Here's how the part is built. I have some questions about the finished solid (model axes, mm). Coordinates: 2 decimals unless noted, no trailing zeros. Write each loop counter-clockwise with the first axis right and the second up, starting at its lowest first coordinate (ties: lowest second). Pieces come first, ordered by that corner, then holes. Notation, with made-up numbers: (33, 8) -> (63, 8) arc R7 ccw to (63, 13) -> close; hole circle Ø2 at (51, -12.5). An arc over 180 degrees is marked (long way). Use CSV: the item, a comma, the result in double quotes. Start each with the question number.
```python
from build123d import *

# Parameters (mm, degrees)
CUT_EXTRUDE1_DEPTH = 0.8
FILLET1_R          = 0.1
FILLET2_R          = 0.1


with BuildPart() as part:
    # Sketch1 → Revolve1 (revolve)
    with BuildSketch(Plane(origin=(0, 0, 0), x_dir=(0, 0, -1), z_dir=(1, 0, 0)), mode=Mode.PRIVATE) as revolve1_sk:
        with BuildLine():
            Line((0, 0), (7, 0))
            Line((7, 0), (7, 0.95))
            Line((7, 0.95), (1.25, 0.95))
            Line((1.25, 0.95), (1.25, 1.625))
            ThreePointArc((1.25, 1.625), (0.348391423, 1.025275828), (0, 0))
        make_face()
    revolve(revolve1_sk.sketch.rotate(Axis((0, 0, 0), (0, 0, -1)), 90), axis=Axis((0, 0, 0), (0, 0, -1)))

    # Sketch2 → Cut-Extrude1 (cut)
    with BuildSketch(Plane.XY):
        with BuildLine():
            Line((-0.375, -2.059291796), (0.375, -2.059291796))
            Line((0.375, -2.059291796), (0.375, -0.649519053))
            ThreePointArc((0.375, -0.649519053), (0.75, 0), (0.375, 0.649519053))
            Line((0.375, 0.649519053), (0.375, 2.059291796))
            Line((0.375, 2.059291796), (-0.375, 2.059291796))
            Line((-0.375, 2.059291796), (-0.375, 0.649519053))
            ThreePointArc((-0.375, 0.649519053), (-0.75, 0), (-0.375, -0.649519053))
            Line((-0.375, -0.649519053), (-0.375, -2.059291796))
        make_face()
    extrude(amount=-CUT_EXTRUDE1_DEPTH, mode=Mode.SUBTRACT)

    # Fillet1
    fillet1_edges = [part.edges().sort_by_distance(p)[0] for p in [
        (-1.625, 0, -1.25),
    ]]
    fillet(fillet1_edges, radius=FILLET1_R)

    # Fillet2
    fillet2_edges = [part.edges().sort_by_distance(p)[0] for p in [
        (-0.95, 0, -7),
    ]]
    fillet(fillet2_edges, radius=FILLET2_R)


solid = part.part
```
Item 1: I'm going to push a flat-ended pin straight in: pin 1 (1 mm diameter, centred on y = 1, z = -5.5, fed in from -X). Where does the tip first touch, or does it pass through?
Item 2: I want a section at A-A on z = -2.25. Please give me the cut outline in (x, y), then the cut area to 3 significant figures.
Item 3: If I drill on line 1 along Z through (x, y) = (0.65, 0.15); line 2 along Z through (x, y) = (1, -0.8); line 3 along Y through (x, z) = (0.1, -1.75), over which ranges is the centre line in solid material (lowest first)?
Item 4: Thinking about a two-plate mould opening in X: for faces 1 (the cylindrical face through (0.9, -0.3, -4)), 2 (the flat face through (0, 0, -0.8)), 3 (the flat face through (0, 0, -7)), which applies, +X half, -X half, draft (parallel to the pull), parting line (faces both ways), or undercut?
Geometry says:
1,pin 1,"x = -0.81"
2,outline,"circle Ø1.9 at (0, 0)"
2,area,"2.84 mm2"
3,line 1,"-7 to -0.8"
3,line 2,"-1.25 to -0.59"
3,line 3,"-0.94 to 0.94"
4,face 1,"parting line"
4,face 2,"undercut"
4,face 3,"draft"
